Answer from the drawing. Dimensions are ordinates in mm from the lowest x, y and z of the part. A direction names the side the tool comes from. Give positions to 0.01 mm unless a question says otherwise; leave off trailing zeros. Loops run counter-clockwise (first coordinate to the right, second up) from the corner with the lowest first, then second, coordinate; pieces in that order, holes last. Notation, with made-up numbers: (17, 34) - (61, 34) arc R14 ccw to (61, 58) - close; hole circle Ø10 at (5.5, 86). An arc over 180 degrees is marked (long way). One line per item, written item: value.
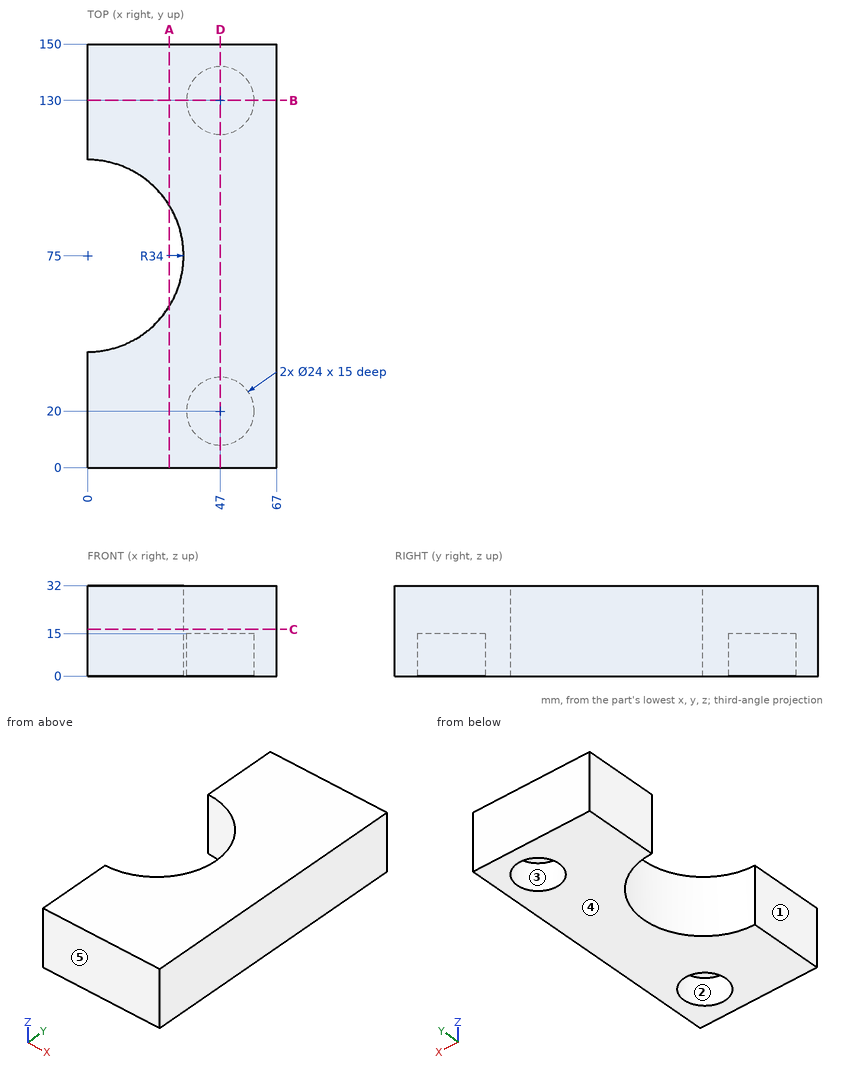
1. Section C-C (z = 16.5) is taken. Write down the section's boundary in (x, y).
Output:
outline: (0, 0) - (67, 0) - (67, 150) - (0, 150) - (0, 109) arc R34 cw to (0, 41) - close
2. The mould has two halves that part along Y. Classify the marked faces 3, 4 and 5: released by +Y, released by -Y, zero draft, split by the parting line, or undercut.
Output:
face 3: undercut
face 4: zero draft
face 5: released by -Y
3. Section D-D (x = 47) is taken. Write down the section's boundary in (y, z), and give its area (3 significant figures).
Output:
outline: (0, 0) - (8, 0) - (8, 15) - (32, 15) - (32, 0) - (118, 0) - (118, 15) - (142, 15) - (142, 0) - (150, 0) - (150, 32) - (0, 32) - close
area: 4,080 mm²
4. Find the intervals of material crossed by line 1 along Y through (x, z) = (47, 11.5); line 2 along Y through (x, z) = (55, 6); line 3 along Y through (x, z) = (6, 6), in increasing order.
Output:
line 1: y = 0 to 8, 32 to 118, 142 to 150
line 2: y = 0 to 11.06, 28.94 to 121.06, 138.94 to 150
line 3: y = 0 to 41.53, 108.47 to 150
5. Section A-A (x = 29) is taken. Write down the section's boundary in (y, z).
Output:
outline: (0, 0) - (57.25, 0) - (57.25, 32) - (0, 32) - close; (92.75, 0) - (150, 0) - (150, 32) - (92.75, 32) - close
6. For the marked faces 1 and 2, determine the directions among +Z, -Z, +X, -X, +Y, -Y from which every point of the face is accessible in a straight line to the end or side of a thin tool.
Output:
face 1: +Z, -Z, -X, +Y, -Y
face 2: -Z
7. Flat-ended cylindrical pins translate along their axes: pin 1 Ø1 at (y, z) = (44, 27.5) entering from -X; pin 2 Ø12 at (y, z) = (95, 11.5) entering from -X; pin 3 Ø12 at (x, y) = (43.5, 16.5) entering from -Z. Find the tip coordinate at first contact, or state that the pin passes through.
Output:
pin 1: stops at x = 12.8
pin 2: stops at x = 21.91
pin 3: stops at z = 15
8. Section B-B (y = 130) is taken. Write down the section's boundary in (x, z), and give its area (3 significant figures).
Output:
outline: (0, 0) - (35, 0) - (35, 15) - (59, 15) - (59, 0) - (67, 0) - (67, 32) - (0, 32) - close
area: 1,780 mm²
